Read the model definition and answer for the solid it produces. Units are mm, in the model's axes. Coordinates: 2 decimals unless noted, no trailing zeros. Order: outer loops, then holes, each group sorted by start corner. A loop starts at its lowest first (then second) coordinate and runs counter-clockwise, first axis right, second up. Notation, with made-up numbers: M -2.5,-22.5 L 4.5,-22.5 A23 cw 4.5,11.5 Z; hole C 87.25,-17 d4. An arc over 180 degrees is marked long. Put each result on its own line as item: value.
from build123d import *

# Parameters (mm, degrees)
BASPROSKE_W         = 4
BASPROSKE_H         = 6
TOOTHCUT_DEPTH      = 10.38083152
TEETHCUTS_COUNT     = 10
TEETHCUTS_ANGLE     = 324
BORSKE_R            = 2.5
BORE_DEPTH          = 50.0000508
SKETCH2_R           = 3
CUT_EXTRUDE1_DEPTH  = 10.217922092
BOSS_EXTRUDE1_START = -4
SKETCH1_R           = 3
BOSS_EXTRUDE1_DEPTH = 4


with BuildPart() as part:
    # BasProSke → Base-Revolve (revolve)
    with BuildSketch(Plane(origin=(0, 0, 0), x_dir=(1, 0, 0), z_dir=(0, 1, 0)), mode=Mode.PRIVATE) as base_revolve_sk:
        with Locations((2, 3)):
            Rectangle(BASPROSKE_W, BASPROSKE_H)
    revolve(base_revolve_sk.sketch.rotate(Axis((-10, 0, 0), (1, 0, 0)), 180), axis=Axis((-10, 0, 0), (1, 0, 0)))

    # TooCutSke → ToothCut (cut, through all)
    with BuildSketch(Plane(origin=(0, 0, 0), x_dir=(0, 0, -1), z_dir=(1, 0, 0))):
        with BuildLine():
            ThreePointArc((0.59278292, 3.701838653), (0, 3.749), (-0.59278292, 3.701838653))
            ThreePointArc((-0.59278292, 3.701838653), (-0.846593509, 4.924114224), (-1.775771316, 5.757784417))
            ThreePointArc((-1.775771316, 5.757784417), (0, 6.0254), (1.775771316, 5.757784417))
            ThreePointArc((1.775771316, 5.757784417), (0.846593509, 4.924114224), (0.59278292, 3.701838653))
        make_face()
    toothcut = extrude(amount=TOOTHCUT_DEPTH, mode=Mode.SUBTRACT)

    # TeethCuts: ToothCut ×10 about axis
    teethcuts_axis = Axis((-10, 0, 0), (1, 0, 0))
    for i in range(1, TEETHCUTS_COUNT):
        add(toothcut.rotate(teethcuts_axis, i * TEETHCUTS_ANGLE / (TEETHCUTS_COUNT - 1)), mode=Mode.SUBTRACT)

    # BorSke → Bore (cut, symmetric)
    with BuildSketch(Plane(origin=(0, 0, 0), x_dir=(0, 0, -1), z_dir=(1, 0, 0))):
        with Locations(Location((0, 0, 0), (0, 0, 180))):
            Circle(BORSKE_R)
    extrude(amount=BORE_DEPTH, both=True, mode=Mode.SUBTRACT)

    # Sketch2 → Cut-Extrude1 (cut, through all)
    with BuildSketch(Plane.ZY):
        Circle(SKETCH2_R)
    extrude(amount=-CUT_EXTRUDE1_DEPTH, mode=Mode.SUBTRACT)

    # Sketch1 → Boss-Extrude1 (add)
    with BuildSketch(Plane(origin=(4, 0, 0), x_dir=(0, 0, -1), z_dir=(1, 0, 0)).offset(BOSS_EXTRUDE1_START)):
        Circle(SKETCH1_R)
        with BuildLine():
            Line((-0.433026392, -1.678537501), (-0.149160433, -2.514010972))
            ThreePointArc((-0.149160433, -2.514010972), (0.309918975, -2.490426475), (0.756919525, -2.383185438))
            Line((0.756919525, -2.383185438), (0.851603533, -2.351014977))
            ThreePointArc((0.851603533, -2.351014977), (1.271412306, -2.163743179), (1.649835725, -1.902772209))
            Line((1.649835725, -1.902772209), (1.365969766, -1.067298739))
            ThreePointArc((1.365969766, -1.067298739), (1.390891529, -0.685427668), (1.678537501, -0.433026392))
            Line((1.678537501, -0.433026392), (2.514010972, -0.149160433))
            ThreePointArc((2.514010972, -0.149160433), (2.490426475, 0.309918975), (2.383185438, 0.756919525))
            Line((2.383185438, 0.756919525), (2.351014977, 0.851603533))
            ThreePointArc((2.351014977, 0.851603533), (2.163743179, 1.271412306), (1.902772209, 1.649835725))
            Line((1.902772209, 1.649835725), (1.067298739, 1.365969766))
            ThreePointArc((1.067298739, 1.365969766), (0.685427668, 1.390891529), (0.433026392, 1.678537501))
            Line((0.433026392, 1.678537501), (0.149160433, 2.514010972))
            ThreePointArc((0.149160433, 2.514010972), (-0.309918975, 2.490426475), (-0.756919525, 2.383185438))
            Line((-0.756919525, 2.383185438), (-0.851603533, 2.351014977))
            ThreePointArc((-0.851603533, 2.351014977), (-1.271412306, 2.163743179), (-1.649835725, 1.902772209))
            Line((-1.649835725, 1.902772209), (-1.365969766, 1.067298739))
            ThreePointArc((-1.365969766, 1.067298739), (-1.390891529, 0.685427668), (-1.678537501, 0.433026392))
            Line((-1.678537501, 0.433026392), (-2.514010972, 0.149160433))
            ThreePointArc((-2.514010972, 0.149160433), (-2.490426475, -0.309918975), (-2.383185438, -0.756919525))
            Line((-2.383185438, -0.756919525), (-2.351014977, -0.851603533))
            ThreePointArc((-2.351014977, -0.851603533), (-2.163743179, -1.271412306), (-1.902772209, -1.649835725))
            Line((-1.902772209, -1.649835725), (-1.067298739, -1.365969766))
            ThreePointArc((-1.067298739, -1.365969766), (-0.685427668, -1.390891529), (-0.433026392, -1.678537501))
        make_face(mode=Mode.SUBTRACT)
    extrude(amount=BOSS_EXTRUDE1_DEPTH)


solid = part.part
Q1. Find section C-C on z = 0. Write down the section's boundary in (x, y).
Answers below:
outline: M 0,-3.75 L 4,-3.75 L 4,-2.52 L 0,-2.52 Z; M 0,2.52 L 4,2.52 L 4,3.75 L 0,3.75 Z
Q2. Find section A-A on y = 4.5. Write down the section's boundary in (x, z), plus the area to 3 significant figures.
Answers below:
outline: M 0,-2.21 L 4,-2.21 L 4,-0.66 L 0,-0.66 Z; M 0,0.66 L 4,0.66 L 4,2.21 L 0,2.21 Z
area: 12.4 mm^2
Q3. Given pin 1 (2 mm diameter, centred on x = 0.5, y = 4, fed in from +Z); pin 2 (2 mm diameter, centred on x = 1.5, z = -0.5, fed in from -Y), each flat-ended and moving along its own axis, determine where each tip first touches the part or whether it passes through.
Answers below:
pin 1: stops at z = 4.92
pin 2: stops at y = -5.61
Q4. Find section B-B on z = -3.5. Write down the section's boundary in (x, y).
Answers below:
outline: M 0,-3.45 L 4,-3.45 L 4,-1.75 L 0,-1.75 Z; M 0,-1.34 L 4,-1.34 L 4,1.34 L 0,1.34 Z; M 0,1.75 L 4,1.75 L 4,3.45 L 0,3.45 Z
Q5. Consider line 1 along Z through (x, y) = (0.3, 0); line 2 along Y through (x, z) = (3.3, 4.25); line 3 along Z through (x, y) = (2.3, -3.5). Determine where each line is inside the solid, lowest interval first.
Answers below:
line 1: z = -6 to -2.52, 2.52 to 6
line 2: y = -3.65 to -2.16, -0.74 to 0.74, 2.16 to 3.65
line 3: z = -4.87 to -3.61, -1.83 to 1.83, 3.61 to 4.87
Q6. Find section D-D on z = 3. Write down the section's boundary in (x, y).
Answers below:
outline: M 0,-3.09 L 4,-3.09 L 4,3.09 L 0,3.09 Z
Q7. For a pull along Z with two mould halves and no side action, classify faces 1 (the face through (1.972, 3.471, 3.546)), 2 (the face through (1.972, -0.724, -4.909)) as +Z half, -Z half, draft (parallel to the pull), parting line (faces both ways), or undercut.
Answers below:
face 1: undercut
face 2: undercut
